from build123d import *

# Parameters (mm, degrees)
BOSS_EXTRU_1_DEPTH = 2.8
CONG_1_R           = 0.6


with BuildPart() as part:
    # Esquisse1 → Boss.-Extru.1 (new body)
    with BuildSketch(Plane.XY):
        with BuildLine():
            Line((-47.370877129, 16), (-34.870877129, 16))
            Line((-34.870877129, 16), (-34.870877129, 12))
            Line((-34.870877129, 12), (-32.570877129, 12))
            Line((-32.570877129, 12), (-32.570877129, 16))
            Line((-32.570877129, 16), (-6.970877129, 16))
            Line((-6.970877129, 16), (-6.970877129, 12))
            Line((-6.970877129, 12), (-4.670877129, 12))
            Line((-4.670877129, 12), (-4.670877129, 16))
            Line((-4.670877129, 16), (-0.670877129, 16))
            ThreePointArc((-0.670877129, 16), (-3.3, 0), (-0.670877129, -16))
            Line((-0.670877129, -16), (-4.670877129, -16))
            Line((-4.670877129, -16), (-4.670877129, -12))
            Line((-4.670877129, -12), (-6.970877129, -12))
            Line((-6.970877129, -12), (-6.970877129, -16))
            Line((-6.970877129, -16), (-32.570877129, -16))
            Line((-32.570877129, -16), (-32.570877129, -12))
            Line((-32.570877129, -12), (-34.870877129, -12))
            Line((-34.870877129, -12), (-34.870877129, -16))
            Line((-34.870877129, -16), (-47.370877129, -16))
            ThreePointArc((-47.370877129, -16), (-50, 0), (-47.370877129, 16))
        make_face()
    extrude(amount=BOSS_EXTRU_1_DEPTH)

    # Congé1
    cong_1_edges = [part.edges().sort_by_distance(p)[0] for p in [
        (-34.870877129, -14, 2.8),
        (-33.720877129, -12, 2.8),
        (-32.570877129, -14, 2.8),
        (-41.120877129, 16, 0),
        (-34.870877129, 14, 0),
        (-33.720877129, 12, 0),
        (-32.570877129, 14, 0),
        (-19.770877129, 16, 0),
        (-19.770877129, -16, 2.8),
        (-6.970877129, 14, 0),
        (-5.820877129, 12, 0),
        (-4.670877129, 14, 0),
        (-2.670877129, 16, 0),
        (-3.3, 0, 0),
        (-2.670877129, -16, 0),
        (-4.670877129, -14, 0),
        (-6.970877129, -14, 2.8),
        (-5.820877129, -12, 0),
        (-6.970877129, -14, 0),
        (-19.770877129, -16, 0),
        (-32.570877129, -14, 0),
        (-33.720877129, -12, 0),
        (-34.870877129, -14, 0),
        (-41.120877129, -16, 0),
        (-50, 0, 0),
        (-5.820877129, -12, 2.8),
        (-4.670877129, -14, 2.8),
        (-2.670877129, -16, 2.8),
        (-47.370877129, 16, 1.4),
        (-34.870877129, 16, 1.4),
        (-32.570877129, 16, 1.4),
        (-6.970877129, 16, 1.4),
        (-4.670877129, 16, 1.4),
        (-0.670877129, 16, 1.4),
        (-0.670877129, -16, 1.4),
        (-4.670877129, -16, 1.4),
        (-6.970877129, -16, 1.4),
        (-32.570877129, -16, 1.4),
        (-34.870877129, -16, 1.4),
        (-47.370877129, -16, 1.4),
        (-3.3, 0, 2.8),
        (-2.670877129, 16, 2.8),
        (-50, 0, 2.8),
        (-4.670877129, 14, 2.8),
        (-5.820877129, 12, 2.8),
        (-6.970877129, 14, 2.8),
        (-19.770877129, 16, 2.8),
        (-32.570877129, 14, 2.8),
        (-33.720877129, 12, 2.8),
        (-34.870877129, 14, 2.8),
        (-41.120877129, 16, 2.8),
        (-41.120877129, -16, 2.8),
    ]]
    fillet(cong_1_edges, radius=CONG_1_R)


solid = part.part
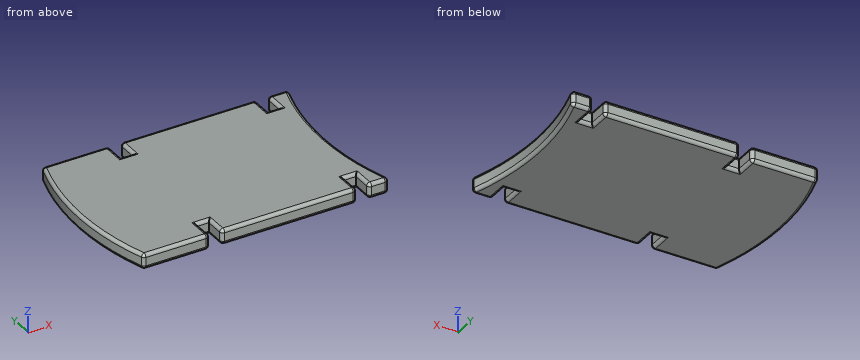
Work out the finished part from the listing and answer in its coordinate system (mm). Give positions to 0.01 mm unless a question says otherwise; leave off trailing zeros. Order: outer loops, then holes, each group sorted by start corner. A loop starts at its lowest first (then second) coordinate and runs counter-clockwise, first axis right, second up. Notation, with made-up numbers: M 38.25,74 L 67.25,74 A9 ccw 67.25,78 Z; hole C 25,5 d3. An arc over 180 degrees is marked long. Return JSON: item names as keys, results as strings.
Q1. Find the intervals of material crossed by line 1 along X through (y, z) = (-0.5, 1); line 2 along X through (y, z) = (-15, 0.85); line 3 along Y through (x, z) = (-38.5, 0.5), in increasing order. Write a range as [from, to].
Answer below:
{"line 1": "x = [-50, -3.3]", "line 2": "x = [-47.7, -34.87], [-32.57, -6.97], [-4.67, -1]", "line 3": "y = [-15.99, 15.99]"}
Q2. Each of these flat-tipped pins is pushed along its axis until it touches: pin 1 (1.5 mm diameter, centred on y = 0.5, z = 1, fed in from +X); pin 2 (1.3 mm diameter, centred on x = -34, z = 1.5, fed in from -Y); pin 3 (0.8 mm diameter, centred on y = -13, z = 1, fed in from +X). Where does it stop, or does it pass through?
Answer below:
{"pin 1": "stops at x = -3.28", "pin 2": "stops at y = -12", "pin 3": "stops at x = -1.47"}
Q3. Find section A-A, the plane x = -34. Write down the section's boundary in (y, z).
Answer below:
{"outline": "M -12,0.6 A0.6 ccw -11.4,0 L 11.4,0 A0.6 ccw 12,0.6 L 12,2.2 A0.6 ccw 11.4,2.8 L -11.4,2.8 A0.6 ccw -12,2.2 Z"}
